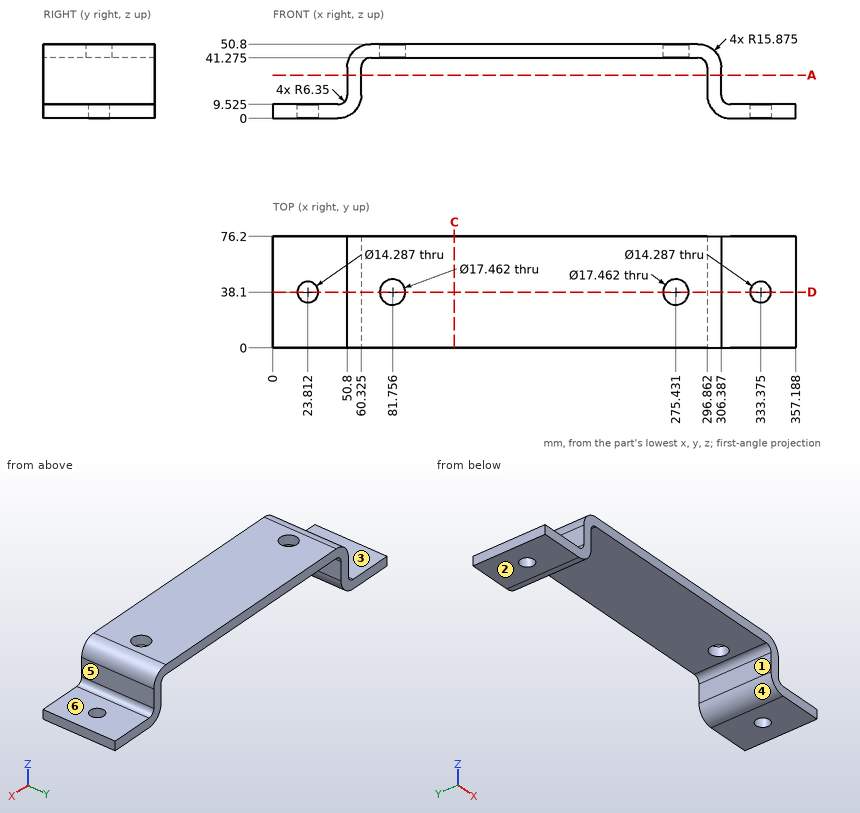
The drawing under review shows one solid part. Ordinate dimensions are in mm from its lowest x, y, z. A direction names the side the tool comes from. Coordinates: 2 decimals unless noted, no trailing zeros. Order: outer loops, then holes, each group sorted by start corner. A loop starts at its lowest first (then second) coordinate and runs counter-clockwise, first axis right, second up. Notation, with made-up numbers: (-9, 37) -> (12, 37) arc R23 cw to (12, 64) -> close; hole circle Ø8 at (88, 66.5). An arc over 180 degrees is marked (long way). Answer in a Markdown table with one row per item.
(1) Consider section D-D (y = 38.1). State how many separate pieces and enclosed holes the cut face has, plus the area to 3 significant figures.
Answers:
| item | result |
|---|---|
| separate pieces | 5 |
| enclosed holes | 0 |
| area | 3,400 mm² |
(2) Consider section A-A (z = 29.5). Write out the cut boundary in (x, y) (1 decimal), plus the area to 3 significant figures.
Answers:
| item | result |
|---|---|
| outline | (50.8, 0) -> (60.3, 0) -> (60.3, 76.2) -> (50.8, 76.2) -> close; (296.9, 0) -> (306.4, 0) -> (306.4, 76.2) -> (296.9, 76.2) -> close |
| area | 1,450 mm² |
(3) Insertion check: pin 1 (9.5 mm diameter, centred on y = 33.5, z = 26, fed in from -X); pin 2 (3 mm diameter, centred on x = 166.5, y = 49, fed in from -Z) (1 decimal); pin 3 (22 mm diameter, centred on x = 19, y = 26.5, fed in from +Z) (1 decimal). Each pin has a flat end and moves straight along its axis. Give the tip position at first contact, or say it passes through.
Answers:
| item | result |
|---|---|
| pin 1 | x = 50.8 |
| pin 2 | z = 41.3 |
| pin 3 | z = 9.5 |
(4) Consider section C-C (x = 124). Write out the cut boundary in (y, z) (1 decimal), plus the area to 3 significant figures.
Answers:
| item | result |
|---|---|
| outline | (0, 41.3) -> (76.2, 41.3) -> (76.2, 50.8) -> (0, 50.8) -> close |
| area | 726 mm² |
(5) The part is to be moulded in two halves that separate along X. For the marked faces 4, 5 and 6, say which applies: +X half, -X half, draft (parallel to the pull), parting line (faces both ways), or undercut.
Answers:
| item | result |
|---|---|
| face 4 | undercut |
| face 5 | +X half |
| face 6 | draft |
(6) Wall thickness on line 1 along X through (y, z) = (38, 2) (1 decimal); line 2 along X through (y, z) = (48.5, 26) (1 decimal); line 3 along X through (y, z) = (15.5, 15): over which ranges is each line inside the solid? List them lowest first.
Answers:
| item | result |
|---|---|
| line 1 | 0 to 16.7, 31 to 52.2, 305 to 326.2, 340.5 to 357.2 |
| line 2 | 50.8 to 60.3, 296.9 to 306.4 |
| line 3 | 50.74 to 60.3, 296.89 to 306.45 |
(7) Machinability: for the marked faces 1, 2 and 3, which of the approach directions +Z, -Z, +X, -X, +Y, -Y give a long, thin tool a straight path to every point of the face, cutting with its end or side? Answer none if there is none.
Answers:
| item | result |
|---|---|
| face 1 | -Z, +Y, -Y |
| face 2 | -Z, +X, -X, +Y, -Y |
| face 3 | +Z, -X, +Y, -Y |
